Part model, mm, in its own coordinate system. A direction names the side the tool comes from. Coordinates: 2 decimals unless noted, no trailing zeros. Write each loop counter-clockwise with the first axis right and the second up, starting at its lowest first coordinate (ties: lowest second). Pieces come first, ordered by that corner, then holes. Notation, with made-up numbers: (9, 28.5) - (52, 28.5) arc R19 ccw to (52, 41.5) - close; hole circle Ø4 at (55, 60.25). An arc over 180 degrees is marked (long way). Use a Markdown table: item, result.
```python
from build123d import *

# Parameters (mm, degrees)
SKETCH_1_W          = 38
SKETCH_1_H          = 38
EXTRUDE_1_DEPTH     = 1.5
SKETCH_2_R          = 1
CUT_EXTRUDE_1_DEPTH = 1.5
SKETCH_3_W          = 10
SKETCH_3_H          = 4
EXTRUDE_2_DEPTH     = 7
SKETCH_4_W          = 9.5
SKETCH_4_H          = 3.5
CUT_EXTRUDE_4_DEPTH = 5
SKETCH_6_R          = 1
CUT_EXTRUDE_6_DEPTH = 10


with BuildPart() as part:
    # 草图1 → 凸台-拉伸1 (new body)
    with BuildSketch(Plane(origin=(0, 0, 0), x_dir=(0, 0, -1), z_dir=(1, 0, 0))):
        Rectangle(SKETCH_1_W, SKETCH_1_H)
    extrude(amount=EXTRUDE_1_DEPTH)

    # 草图2 → 切除-拉伸1 (cut)
    with BuildSketch(Plane(origin=(1.5, 0, 0), x_dir=(0, 0, -1), z_dir=(1, 0, 0))):
        with Locations((-14, 14)):
            Circle(SKETCH_2_R)
        with Locations((-14, -14)):
            Circle(SKETCH_2_R)
        with Locations((14, -14)):
            Circle(SKETCH_2_R)
        with Locations((14, 14)):
            Circle(SKETCH_2_R)
        with Locations((-12.5, 0)):
            Circle(SKETCH_2_R)
        with Locations((12.5, 0)):
            Circle(SKETCH_2_R)
    extrude(amount=-CUT_EXTRUDE_1_DEPTH, mode=Mode.SUBTRACT)

    # 草图3 → 凸台-拉伸2 (add)
    with BuildSketch(Plane.ZY):
        with Locations((-5.878697065, 12.867552656)):
            Rectangle(SKETCH_3_W, SKETCH_3_H)
    extrude(amount=EXTRUDE_2_DEPTH)

    # 草图4 → 切除-拉伸4 (cut)
    with BuildSketch(Plane.ZY.offset(7)):
        with Locations((-5.878697065, 12.867552656)):
            Rectangle(SKETCH_4_W, SKETCH_4_H)
    extrude(amount=-CUT_EXTRUDE_4_DEPTH, mode=Mode.SUBTRACT)

    # 草图6 → 切除-拉伸6 (cut)
    with BuildSketch(Plane(origin=(1.5, 0, 0), x_dir=(0, 0, -1), z_dir=(1, 0, 0))):
        with Locations((-9, 0)):
            Circle(SKETCH_6_R)
        with Locations((9, 0)):
            Circle(SKETCH_6_R)
    extrude(amount=-CUT_EXTRUDE_6_DEPTH, mode=Mode.SUBTRACT)


solid = part.part
```
Item 1: Band-saw the part on A-A, the plane z = -12.5. Give the cut face in (x, y).
From the geometry:
| item | result |
|---|---|
| outline | (0, -19) - (1.5, -19) - (1.5, -1) - (0, -1) - close; (0, 1) - (1.5, 1) - (1.5, 19) - (0, 19) - close |
Item 2: Band-saw the part on C-C, the plane x = -2.5. Give the cut face in (y, z), then the cut area to 3 significant figures.
From the geometry:
| item | result |
|---|---|
| outline | (10.87, -10.88) - (14.87, -10.88) - (14.87, -0.88) - (10.87, -0.88) - close; hole (11.12, -10.63) - (14.62, -10.63) - (14.62, -1.13) - (11.12, -1.13) - close |
| area | 6.75 mm^2 |
Item 3: Band-saw the part on B-B, the plane y = 0. Give the cut face in (x, z).
From the geometry:
| item | result |
|---|---|
| outline | (0, -19) - (1.5, -19) - (1.5, -13.5) - (0, -13.5) - close; (0, -11.5) - (1.5, -11.5) - (1.5, -10) - (0, -10) - close; (0, -8) - (1.5, -8) - (1.5, 8) - (0, 8) - close; (0, 10) - (1.5, 10) - (1.5, 11.5) - (0, 11.5) - close; (0, 13.5) - (1.5, 13.5) - (1.5, 19) - (0, 19) - close |
Item 4: Which spindle directions (+Z, -Z, +X, -X, +Y, -Y) get a long thin tool onto all of the face, cutting with end or side? Do faces 1 (the face through (-3, 10.868, -6)), 2 (the face through (-2, 13, -6)), 3 (the face through (-3, 13, -10.879)), 4 (the face through (0.8, 0, -11.5)). Say none if no direction does.
From the geometry:
| item | result |
|---|---|
| face 1 | +Z, -Z, -X, -Y |
| face 2 | -X |
| face 3 | -Z, -X, +Y, -Y |
| face 4 | +X, -X |
Item 5: Band-saw the part on D-D, the plane y = -14. Give the cut face in (x, z).
From the geometry:
| item | result |
|---|---|
| outline | (0, -19) - (1.5, -19) - (1.5, -15) - (0, -15) - close; (0, -13) - (1.5, -13) - (1.5, 13) - (0, 13) - close; (0, 15) - (1.5, 15) - (1.5, 19) - (0, 19) - close |
Item 6: Drop flat-ended pins along their axis: P1, Ø11.5, axis at y = 4.5, z = -3.5, coming from the -X side; P2, Ø1.6, axis at y = 0, z = 9, coming from the +X side; P3, Ø1.8, axis at x = -4.5, y = 12.5, coming from the +Z side; P4, Ø4.5, axis at x = -5, y = 13.5, coming from the -Z side. Give the stop position or say it passes through.
From the geometry:
| item | result |
|---|---|
| P1 | x = 0 |
| P2 | through |
| P3 | z = -0.88 |
| P4 | z = -10.88 |
Item 7: Drill centre lines: probe 1 along Y at (x, z) = (0.8, -14); probe 2 along Y at (x, z) = (-4.25, -8); probe 3 along X at (y, z) = (-16, -3). Where is each one in solid material? Low to high.
From the geometry:
| item | result |
|---|---|
| probe 1 | -19 to -15, -13 to 13, 15 to 19 |
| probe 2 | 10.87 to 11.12, 14.62 to 14.87 |
| probe 3 | 0 to 1.5 |
